from build123d import *

# Parameters (mm, degrees)
BOSS_EXTRU_1_DEPTH      = 430
ENL_V_MAT_EXTRU_1_DEPTH = 453.65881191


with BuildPart() as part:
    # Esquisse2 → Boss.-Extru.1 (new body)
    with BuildSketch(Plane(origin=(0, 0, 0), x_dir=(1, 0, 0), z_dir=(0, 1, 0))):
        with BuildLine():
            Line((2, 0), (98, 0))
            ThreePointArc((98, 0), (99.414213562, 0.585786438), (100, 2))
            Line((100, 2), (100, 98))
            ThreePointArc((100, 98), (99.414213562, 99.414213562), (98, 100))
            Line((98, 100), (2, 100))
            ThreePointArc((2, 100), (0.585786438, 99.414213562), (0, 98))
            Line((0, 98), (0, 2))
            ThreePointArc((0, 2), (0.585786438, 0.585786438), (2, 0))
        make_face()
        with BuildLine():
            Line((6, 96), (94, 96))
            ThreePointArc((94, 96), (95.414213562, 95.414213562), (96, 94))
            Line((96, 94), (96, 6))
            ThreePointArc((96, 6), (95.414213562, 4.585786438), (94, 4))
            Line((94, 4), (6, 4))
            ThreePointArc((6, 4), (4.585786438, 4.585786438), (4, 6))
            Line((4, 6), (4, 94))
            ThreePointArc((4, 94), (4.585786438, 95.414213562), (6, 96))
        make_face(mode=Mode.SUBTRACT)
    extrude(amount=BOSS_EXTRU_1_DEPTH)

    # Esquisse3 → Enlèv. mat.-Extru.1 (cut, through all)
    with BuildSketch(Plane.XY):
        Polygon((45, 430), (0, 352.057713659), (-62.450183936, 352.057713659), (-62.450183936, 486.30167962), (45, 486.30167962), align=None)
        Polygon((45, 0), (0, 77.942286341), (-44.197295574, 77.942286341), (-44.197295574, -11.830713302), (45, -11.830713302), align=None)
        Polygon((55, -11.830713302), (55, 0), (100, 77.942286341), (144.197295574, 77.942286341), (144.197295574, -11.830713302), align=None)
        Polygon((55, 486.30167962), (55, 430), (100, 352.057713659), (162.450183936, 352.057713659), (162.450183936, 486.30167962), align=None)
    extrude(amount=-ENL_V_MAT_EXTRU_1_DEPTH, mode=Mode.SUBTRACT)


solid = part.part
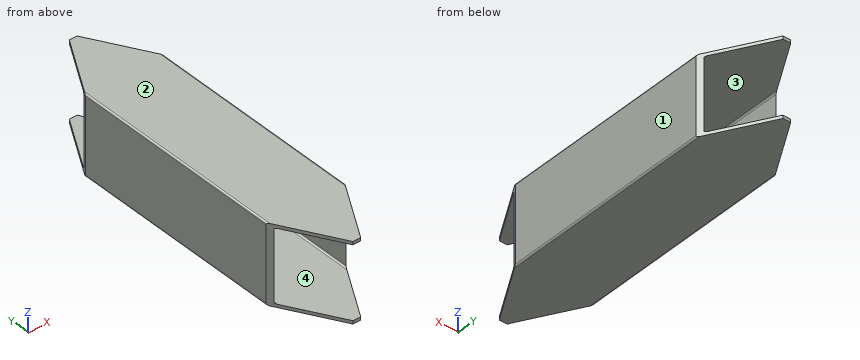
Check sheet for the modelled part. Datum: model origin and axes. Units: mm. Face numbers are marked on the shaded views. Coordinates: 2 decimals unless noted, no trailing zeros. Loops run counter-clockwise (first coordinate to the right, second up) from the corner with the lowest first, then second, coordinate; pieces in that order, holes last. Notation, with made-up numbers: (47, 61.5) -> (86, 61.5) arc R20 cw to (86, 88.5) -> close; hole circle Ø5 at (-30, 48.25). An arc over 180 degrees is marked (long way). Answer in a Markdown table with one row per item.
1. Material ranges on line 1 along Z through (x, y) = (17.5, 182.5); line 2 along X through (y, z) = (90, -37.5); line 3 along X through (y, z) = (75.5, -38.5), recorded low to high. Write a range as [from, to].
Check values:
| item | result |
|---|---|
| line 1 | z = [-100, -96], [-4, 0] |
| line 2 | x = [0, 4], [96, 100] |
| line 3 | x = [1.41, 4], [96, 98.59] |
2. Sectioned sample at C-C, the plane y = 238.5. Record the boundary of the cut face in (x, z).
Check values:
| item | result |
|---|---|
| outline | (0, -98) arc R2 ccw to (2, -100) -> (98, -100) arc R2 ccw to (100, -98) -> (100, -2) arc R2 ccw to (98, 0) -> (2, 0) arc R2 ccw to (0, -2) -> close; hole (4, -94) arc R2 ccw to (6, -96) -> (94, -96) arc R2 ccw to (96, -94) -> (96, -6) arc R2 ccw to (94, -4) -> (6, -4) arc R2 ccw to (4, -6) -> close |
3. Release check for a two-part mould opening along X. For the marked faces 1, 2, 3 and 4 record: released by +X, released by -X, zero draft, split by the parting line, or undercut.
Check values:
| item | result |
|---|---|
| face 1 | released by +X |
| face 2 | zero draft |
| face 3 | undercut |
| face 4 | undercut |
4. Sectioned sample at A-A, the plane y = 396. Record the boundary of the cut face in (x, z), then the cut area to 3 significant figures.
Check values:
| item | result |
|---|---|
| outline | (25.37, -100) -> (74.63, -100) -> (74.63, -96) -> (25.37, -96) -> close; (25.37, -4) -> (74.63, -4) -> (74.63, 0) -> (25.37, 0) -> close |
| area | 394 mm2 |
5. Sectioned sample at B-B, the plane z = -23.5. Record the boundary of the cut face in (x, y), then the cut area to 3 significant figures.
Check values:
| item | result |
|---|---|
| outline | (0, 77.94) -> (4, 71.01) -> (4, 358.99) -> (0, 352.06) -> close; (96, 71.01) -> (100, 77.94) -> (100, 352.06) -> (96, 358.99) -> close |
| area | 2,250 mm2 |
